Part model, mm, in its own coordinate system. Face numbers are marked on the shaded views. A direction names the side the tool comes from. Round coordinates to 2 decimals unless told otherwise and drop trailing zeros. Order: outer loops, then holes, each group sorted by start corner. A loop starts at its lowest first (then second) coordinate and runs counter-clockwise, first axis right, second up. Notation, with made-up numbers: M -16.5,-14.5 L 23.5,-14.5 A16 cw 23.5,-7.5 Z; hole C 36.25,24 d11. An arc over 180 degrees is marked long. One line per question, with ' | ' between items.
from build123d import *

# Parameters (mm, degrees)
F1_DEPTH  = 1
F3_DEPTH  = 1
F10_R     = 1
F11_DEPTH = 25


with BuildPart() as f1:
    # F0 (on Front) → F1 (new body)
    with BuildSketch(Plane.XZ):
        with BuildLine():
            Line((0, -25), (-31.224989992, -25))
            ThreePointArc((-31.224989992, -25), (-28.2842712475, -28.2842712475), (-25, -31.224989992))
            Line((-25, -31.224989992), (-25, -40))
            Line((-25, -40), (-15, -40))
            Line((-15, -40), (-15, -37.0809924355))
            ThreePointArc((-15, -37.0809924355), (0, -40), (15, -37.0809924355))
            Line((15, -37.0809924355), (15, -40))
            Line((15, -40), (25, -40))
            Line((25, -40), (25, -31.224989992))
            ThreePointArc((25, -31.224989992), (28.2842712475, -28.2842712475), (31.224989992, -25))
            Line((31.224989992, -25), (0, -25))
        make_face()
    extrude(amount=F1_DEPTH)

    # F2 (on face) → F3 (join)
    with BuildSketch(Plane.XZ.offset(1)):
        with BuildLine():
            Line((5, -25), (0, -25))
            Line((0, -25), (-5, -25))
            Line((-5, -25), (-5, -39.686269666))
            ThreePointArc((-5, -39.686269666), (0, -40), (5, -39.686269666))
            Line((5, -39.686269666), (5, -25))
        make_face()
    extrude(amount=F3_DEPTH)

    # F4 (on face) → F7 section 0
    with BuildSketch(Plane.XZ.offset(2)):
        with BuildLine():
            add(Edge.make_bspline(
                [(4, -36), (4, -32.5358983849), (-2, -34.2679491924), (-8, -36), (-2, -37.7320508076), (4, -39.4641016151), (4, -36)],
                knots=[0, 0, 0, 2.0943951024, 2.0943951024, 4.1887902048, 4.1887902048, 6.2831853072, 6.2831853072, 6.2831853072], degree=2, weights=[1, 0.5, 1, 0.5, 1, 0.5, 1]))
        make_face()
    # F6 (on offset) → F7 section 1
    with BuildSketch(Plane.XZ.offset(32)):
        with BuildLine():
            add(Edge.make_bspline(
                [(2, -36), (2, -34.2679491924), (-1, -35.1339745962), (-4, -36), (-1, -36.8660254038), (2, -37.7320508076), (2, -36)],
                knots=[0, 0, 0, 2.0943951024, 2.0943951024, 4.1887902048, 4.1887902048, 6.2831853072, 6.2831853072, 6.2831853072], degree=2, weights=[1, 0.5, 1, 0.5, 1, 0.5, 1]))
        make_face()
    loft()

    # F8 (on face) → F9 (revolve)
    with BuildSketch(Plane.XZ.offset(32)):
        with BuildLine():
            Line((-4, -36), (4, -36))
            ThreePointArc((4, -36), (0, -32), (-4, -36))
        make_face()
    revolve(axis=Axis((0, -32, -36), (1, 0, 0)))

    # F10 (on face) → F11 (cut)
    with BuildSketch(Plane.XZ.offset(2)):
        with Locations((0, -30)):
            Circle(F10_R)
    extrude(amount=-F11_DEPTH, mode=Mode.SUBTRACT)


solid = f1.part
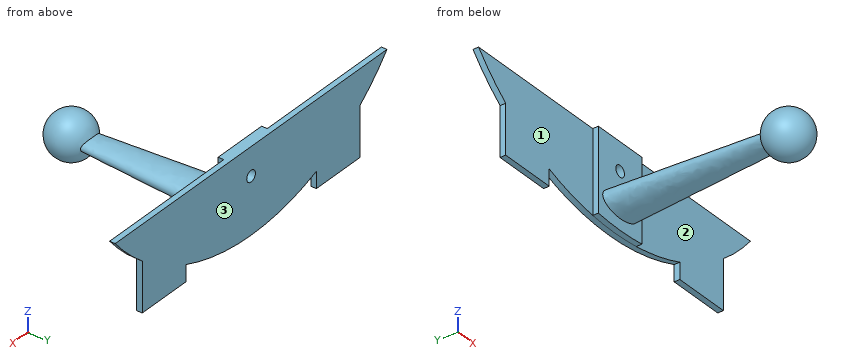
1) Drop flat-ended pins along their axis: pin 1 (1 mm diameter, centred on x = -4.5, z = -34, fed in from +Y); pin 2 (5 mm diameter, centred on x = 1, z = -30.5, fed in from -Y); pin 3 (6 mm diameter, centred on y = -11.5, z = -38, fed in from -X); pin 4 (1.1 mm diameter, centred on y = -0.5, z = -38.5, fed in from -X). Give the stop position or say it passes through.
The answers:
pin 1: stops at y = 0 | pin 2: stops at y = -34.54 | pin 3: stops at x = -3.52 | pin 4: stops at x = -25
2) Saw through at B-B (x = -23.5). List the corners of the cut face in (y, z), plus the area to 3 significant figures.
The answers:
outline: M -1,-40 L 0,-40 L 0,-25 L -1,-25 Z | area: 15.0 mm²
3) Saw through at C-C (x = 9.5). List the corners of the cut face in (y, z).
The answers:
outline: M -1,-38.86 L 0,-38.86 L 0,-25 L -1,-25 Z
4) Saw through at A-A (z = -30). List the corners of the cut face in (x, y), plus the area to 3 significant figures.
The answers:
outline: M -26.46,-1 L -5,-1 L -5,-2 L -1,-2 L -1,0 L -26.46,0 Z; M 1,-2 L 5,-2 L 5,-1 L 26.46,-1 L 26.46,0 L 1,0 Z | area: 58.9 mm²
5) Which spindle directions (+Z, -Z, +X, -X, +Y, -Y) get a long thin tool onto all of the face, cutting with end or side? Do the marked faces 1, 2 and 3. Say none if no direction does.
The answers:
face 1: +Z, -Z, -X, -Y | face 2: +Z, -Z, +X, -Y | face 3: +Z, -Z, +X, -X, +Y
6) Probe line 1 (Z direction, x = 0, y = -1.25); line 2 (Y direction, x = 4.5, z = -31.75); line 3 (Y direction, x = 12, z = -35.75). List the from-to ranges inside material, lowest first. Write a range as [from, to].
The answers:
line 1: z = [-40, -31], [-29, -25] | line 2: y = [-2, 0] | line 3: y = [-1, 0]
